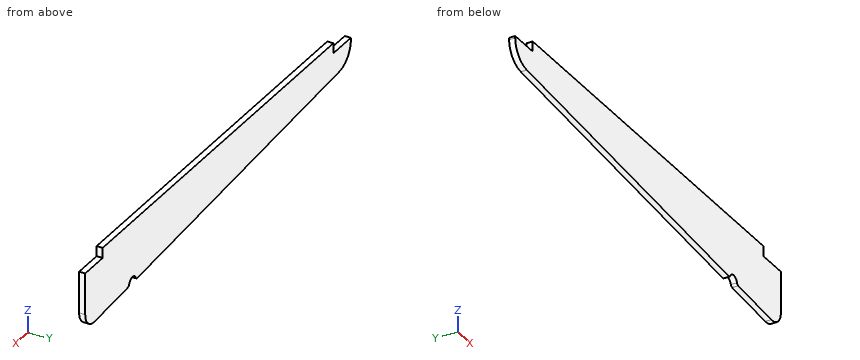
Autodesk Inventor part; units mm, degrees
ref_plane "YZ Plane" through (0, 0, 0) normal (1, 0, 0) x (0, 1, 0)
ref_plane "XZ Plane" through (0, 0, 0) normal (0, 1, 0) x (-1, 0, 0)
ref_plane "XY Plane" through (0, 0, 0) normal (0, 0, 1) x (1, 0, 0)
sketch "Sketch2" plane through (0, 0, 0) normal (0, 1, 0) x (-1, 0, 0)
  line L0 (0, 0) -> (-228, 0)
  line L1 (-228, 0) -> (-228, -33.6943)
  line L2 (-228, -33.6943) -> (0, -16)
  arc A0 (-228, -25.5205) -> (-219.8507, -33.0618) centre (-220.436, -25.5205) ccw
  arc A1 (-184.5652, -29.4637) -> (-190.2978, -29.9086) centre (-187.3652, -30.5408) ccw
  arc A2 (-191.378, -30.8522) -> (-190.2978, -29.9086) centre (-191.4709, -29.6558) ccw
  arc A3 (-184.5652, -29.4637) -> (-183.3523, -30.2293) centre (-183.4452, -29.0329) ccw
  line L3 (0, 0) -> (-15, 0)
  line L4 (-15, 0) -> (-15, -5)
  line L5 (-15, -5) -> (0, -5)
  line L6 (-228, 0) -> (-213, 0)
  line L7 (-213, 0) -> (-213, -5)
  line L8 (-213, -5) -> (-228, -5)
  line L9 (-228, -5) -> (-228, 0)
  line L10 (0, -16) -> (0, -5)
  arc A4 (-9.97, -16.7737) -> (0, -6) centre (-10.8061, -6) ccw
  point P0 (-220.5, -5)
  point P1 (-7.5, -5)
  point P2 (-15, 0)
  dimension "xp" = 228
  dimension "corner" = 7.564
  dimension "d9" = 1.2
  dimension "d10" = 1.2
  dimension "d15" = 15
  dimension "d16" = 3
  dimension "d20" = 15
  dimension "cutoutdepth" = 5
  dimension "cutoutlength" = 198
  dimension "theta" = 4.438
  dimension "raised" = 11
  dimension "d25" = 10.8061
  dimension "d26" = 1
extrude "Extrusion1" add sketch "Sketch2" along normal blind 3 contours L4 L5 L10 A4 L2 A3 A1 A2 A0 L1 L8 L7 L0
equation "\"d15\" = cutoutoffset"
equation "\"d20\" = cutoutoffset"
equation "\"b\" = 17.7"
properties part number "rail"
Read the model definition and answer for the solid it produces. Units are mm, in the model's axes. Give positions to 0.01 mm unless a question says otherwise; leave off trailing zeros. Order: outer loops, then holes, each group sorted by start corner. A loop starts at its lowest first (then second) coordinate and runs counter-clockwise, first axis right, second up.
(1) Find section A-A (y = 2.45). Give the vertices of the cut face in (x, z), plus the area to 3 significant figures.
(2) Find section C-C (x = 141). Give the vertices of the cut face in (y, z), plus the area to 3 significant figures.
(3) Given pin 1 (1 mm diameter, centred on x = 185, y = 1, fed in from +Z); pin 2 (0.9 mm diameter, centred on x = 6, y = 1.5, fed in from +Z), each flat-ended and moving along its own axis, determine where each tip first touches the part or whether it passes through.
(4) Straight lines are drawn through the part: L1, parallel to X at y = 1.6, z = -3; L2, parallel to Z at x = 115.5, y = 0.6; L3, parallel to Z at x = 84.5, y = 2.3. For each, find the intervals that lie inside material, in ascending order.
(5) Find section B-B (z = -14.5). Give the vertices of the cut face in (x, y).
Result sheet:
1. outline: (0, -6) arc R10.81 ccw to (9.97, -16.77) - (183.35, -30.23) arc R1.2 ccw to (184.57, -29.46) arc R3 cw to (190.3, -29.91) arc R1.2 ccw to (191.38, -30.85) - (219.85, -33.06) arc R7.56 ccw to (228, -25.52) - (228, -5) - (213, -5) - (213, 0) - (15, 0) - (15, -5) - (0, -5) - close
1. area: 5,470 mm2
2. outline: (0, -26.94) - (3, -26.94) - (3, 0) - (0, 0) - close
2. area: 80.8 mm2
3. pin 1: stops at z = 0
3. pin 2: stops at z = -5
4. L1: x = 15 to 213
4. L2: z = -24.96 to 0
4. L3: z = -22.56 to 0
5. outline: (4.13, 0) - (228, 0) - (228, 3) - (4.13, 3) - close
